from build123d import *

# Parameters (mm, degrees)
SKETCH1_R                   = 1.2
BOSS_EXTRUDE1_DEPTH         = 1.4
SKETCH2_R                   = 2.25
CUT_EXTRUDE1_DEPTH          = 1.1
CUT_EXTRUDE1_DRAFT          = -45
SKETCH3_W                   = 12
SKETCH3_H                   = 1.5
BOSS_EXTRUDE2_DEPTH         = 3.5
CIRPATTERN1_COUNT           = 2
CIRPATTERN1_ANGLE           = 90
CIRPATTERN1_COPY_1_SKETCH_R = 2.25
CIRPATTERN1_COPY_1_DEPTH    = 1.1
CIRPATTERN1_COPY_1_DRAFT    = -45
CIRPATTERN2_START           = -14
CIRPATTERN2_OUTLINE_W       = 1.5
CIRPATTERN2_OUTLINE_H       = 3.5
CIRPATTERN2_DEPTH           = 12
CIRPATTERN2_2_OUTLINE_R     = 1.2
CIRPATTERN2_2_DEPTH         = 1.4
CIRPATTERN2_START_2         = -2.1
CIRPATTERN2_3_OUTLINE_W     = 12
CIRPATTERN2_3_OUTLINE_H     = 1.5
CIRPATTERN2_3_DEPTH         = 2.1
CIRPATTERN3_COPY_1_SKETCH_R = 2.25
CIRPATTERN3_COPY_1_DEPTH    = 1.1
CIRPATTERN3_COPY_1_DRAFT    = -45
CIRPATTERN3_COPY_2_SKETCH_R = 2.25
CIRPATTERN3_COPY_2_DEPTH    = 1.1
CIRPATTERN3_COPY_2_DRAFT    = -45
CIRPATTERN3_COPY_3_SKETCH_R = 2.25
CIRPATTERN3_COPY_3_DEPTH    = 1.1
CIRPATTERN3_COPY_3_DRAFT    = -45
CUT_EXTRUDE2_DEPTH          = 3
CIRPATTERN4_COUNT           = 4
FILLET2_R                   = 0.25
CUT_EXTRUDE3_DEPTH          = 32.183489221
CUT_EXTRUDE3_DEPTH_BACK     = 32.183489221
SKETCH5_W                   = 28
SKETCH5_H                   = 28
SKETCH5_W_2                 = 27.7
SKETCH5_H_2                 = 27.7
FILLET3_R                   = 2
FILLET4_R                   = 1.1
CUT_EXTRUDE4_DEPTH          = 31.97184205
CUT_EXTRUDE4_DEPTH_BACK     = 31.97184205
SKETCH6_W                   = 0.1
SKETCH6_H                   = 2.1
CUT_EXTRUDE5_DEPTH          = 31.97184205
CUT_EXTRUDE5_DEPTH_BACK     = 31.97184205
SKETCH7_W                   = 0.1
SKETCH7_H                   = 2.1


# Read off the part's stored shape, not the designer's step: CirPattern2
with BuildPart() as part:
    # Sketch1 → Boss-Extrude1 (new body)
    with BuildSketch(Plane(origin=(0, 0, 0), x_dir=(1, 0, 0), z_dir=(0, 1, 0))):
        Polygon((0, 0), (0, 2), (-6, 2), (-6, -6), (2, -6), (2, 0), align=None)
        with Locations(Location((-2, -2, 0), (0, 0, 270))):
            Circle(SKETCH1_R, mode=Mode.SUBTRACT)
    boss_extrude1 = extrude(amount=BOSS_EXTRUDE1_DEPTH)


with BuildPart() as cut_extrude1_tool:
    # Sketch2 → Cut-Extrude1 (with draft: the straight prism first)
    with BuildSketch(Plane(origin=(0, 1.4, 0), x_dir=(1, 0, 0), z_dir=(0, 1, 0))):
        with Locations((-2, -2)):
            Circle(SKETCH2_R)
    extrude(amount=-CUT_EXTRUDE1_DEPTH)
    # Cut-Extrude1: the draft: its side faces are tilted about the plane it starts from
    cut_extrude1_sides = [cut_extrude1_tool.faces().sort_by_distance(p)[0] for p in [
        (-4.25, 0.85, 2),
    ]]
    draft(cut_extrude1_sides, Plane(origin=(0, 1.4, 0), x_dir=(1, 0, 0), z_dir=(0, 1, 0)), CUT_EXTRUDE1_DRAFT)


with BuildPart() as part_1:
    add(part.part)

    # Cut-Extrude1: cut by cut_extrude1_tool
    add(cut_extrude1_tool.part, mode=Mode.SUBTRACT)

    # Sketch3 → Boss-Extrude2 (add)
    with BuildSketch(Plane(origin=(0, 1.4, 0), x_dir=(1, 0, 0), z_dir=(0, 1, 0))):
        with Locations((8, -0.75)):
            Rectangle(SKETCH3_W, SKETCH3_H)
    boss_extrude2 = extrude(amount=-BOSS_EXTRUDE2_DEPTH)

    # CirPattern1: Boss-Extrude1, Boss-Extrude2 ×2 about axis
    cirpattern1_axis = Axis((8, 0, -8), (0, 1, 0))
    add([boss_extrude1.rotate(cirpattern1_axis, i * CIRPATTERN1_ANGLE / (CIRPATTERN1_COUNT - 1)) for i in range(1, CIRPATTERN1_COUNT)])
    add([boss_extrude2.rotate(cirpattern1_axis, i * CIRPATTERN1_ANGLE / (CIRPATTERN1_COUNT - 1)) for i in range(1, CIRPATTERN1_COUNT)])


with BuildPart() as cirpattern1_copy_1_tool:
    # CirPattern1 copy 1 sketch → CirPattern1 copy 1 (with draft: the straight prism first)
    with BuildSketch(Plane(origin=(16, 1.4, 0), x_dir=(0, 0, -1), z_dir=(0, 1, 0))):
        with Locations((-2, -2)):
            Circle(CIRPATTERN1_COPY_1_SKETCH_R)
    extrude(amount=-CIRPATTERN1_COPY_1_DEPTH)
    # CirPattern1 copy 1: the draft: its side faces are tilted about the plane it starts from
    cirpattern1_copy_1_sides = [cirpattern1_copy_1_tool.faces().sort_by_distance(p)[0] for p in [
        (18, 0.85, 4.25),
    ]]
    draft(cirpattern1_copy_1_sides, Plane(origin=(16, 1.4, 0), x_dir=(0, 0, -1), z_dir=(0, 1, 0)), CIRPATTERN1_COPY_1_DRAFT)


with BuildPart() as part_2:
    add(part_1.part)

    # CirPattern1 copy 1: cut by cirpattern1_copy_1_tool
    add(cirpattern1_copy_1_tool.part, mode=Mode.SUBTRACT)

    # CirPattern2 outline → CirPattern2 (add)
    with BuildSketch(Plane.XY.offset(CIRPATTERN2_START)):
        with Locations((-0.75, -0.35)):
            Rectangle(CIRPATTERN2_OUTLINE_W, CIRPATTERN2_OUTLINE_H)
    extrude(amount=CIRPATTERN2_DEPTH)

    # CirPattern2 2 outline → CirPattern2 2 (add)
    with BuildSketch(Plane(origin=(0, 0, 0), x_dir=(1, 0, 0), z_dir=(0, 1, 0))):
        Polygon((2, 16), (16, 16), (16, 14), (22, 14), (22, 22), (14, 22), (14, 17.5), (2, 17.5), align=None)
        with Locations((18, 18)):
            Circle(CIRPATTERN2_2_OUTLINE_R, mode=Mode.SUBTRACT)
    extrude(amount=CIRPATTERN2_2_DEPTH)

    # CirPattern2 3 outline → CirPattern2 3 (add)
    with BuildSketch(Plane(origin=(0, 0, 0), x_dir=(1, 0, 0), z_dir=(0, 1, 0)).offset(CIRPATTERN2_START_2)):
        with Locations((8, 16.75)):
            Rectangle(CIRPATTERN2_3_OUTLINE_W, CIRPATTERN2_3_OUTLINE_H)
    extrude(amount=CIRPATTERN2_3_DEPTH)

    # CirPattern2 4 outline → CirPattern2 4 (revolve)
    with BuildSketch(Plane(origin=(18, 0, 2), x_dir=(1, 0, 0), z_dir=(0, 0, 1))):
        Polygon((1.2, 1.4), (1.2, 0.35), (2.25, 1.4), align=None)
    revolve(axis=Axis((18, 0, 2), (0, 1, 0)))

    # Mirror1: Boss-Extrude1 across plane
    add(boss_extrude1.mirror(Plane(origin=(0, 0, -8), x_dir=(1, 0, 0), z_dir=(0, 0, -1))))


with BuildPart() as cirpattern3_copy_1_tool:
    # CirPattern3 copy 1 sketch → CirPattern3 copy 1 (with draft: the straight prism first)
    with BuildSketch(Plane(origin=(16, 1.4, 0), x_dir=(0, 0, -1), z_dir=(0, 1, 0))):
        with Locations((-2, -2)):
            Circle(CIRPATTERN3_COPY_1_SKETCH_R)
    extrude(amount=-CIRPATTERN3_COPY_1_DEPTH)
    # CirPattern3 copy 1: the draft: its side faces are tilted about the plane it starts from
    cirpattern3_copy_1_sides = [cirpattern3_copy_1_tool.faces().sort_by_distance(p)[0] for p in [
        (18, 0.85, 4.25),
    ]]
    draft(cirpattern3_copy_1_sides, Plane(origin=(16, 1.4, 0), x_dir=(0, 0, -1), z_dir=(0, 1, 0)), CIRPATTERN3_COPY_1_DRAFT)


with BuildPart() as part_3:
    add(part_2.part)

    # CirPattern3 copy 1: cut by cirpattern3_copy_1_tool
    add(cirpattern3_copy_1_tool.part, mode=Mode.SUBTRACT)


with BuildPart() as cirpattern3_copy_2_tool:
    # CirPattern3 copy 2 sketch → CirPattern3 copy 2 (with draft: the straight prism first)
    with BuildSketch(Plane(origin=(16, 1.4, -16), x_dir=(-1, 0, 0), z_dir=(0, 1, 0))):
        with Locations((-2, -2)):
            Circle(CIRPATTERN3_COPY_2_SKETCH_R)
    extrude(amount=-CIRPATTERN3_COPY_2_DEPTH)
    # CirPattern3 copy 2: the draft: its side faces are tilted about the plane it starts from
    cirpattern3_copy_2_sides = [cirpattern3_copy_2_tool.faces().sort_by_distance(p)[0] for p in [
        (20.25, 0.85, -18),
    ]]
    draft(cirpattern3_copy_2_sides, Plane(origin=(16, 1.4, -16), x_dir=(-1, 0, 0), z_dir=(0, 1, 0)), CIRPATTERN3_COPY_2_DRAFT)


with BuildPart() as part_4:
    add(part_3.part)

    # CirPattern3 copy 2: cut by cirpattern3_copy_2_tool
    add(cirpattern3_copy_2_tool.part, mode=Mode.SUBTRACT)


with BuildPart() as cirpattern3_copy_3_tool:
    # CirPattern3 copy 3 sketch → CirPattern3 copy 3 (with draft: the straight prism first)
    with BuildSketch(Plane(origin=(0, 1.4, -16), x_dir=(0, 0, 1), z_dir=(0, 1, 0))):
        with Locations((-2, -2)):
            Circle(CIRPATTERN3_COPY_3_SKETCH_R)
    extrude(amount=-CIRPATTERN3_COPY_3_DEPTH)
    # CirPattern3 copy 3: the draft: its side faces are tilted about the plane it starts from
    cirpattern3_copy_3_sides = [cirpattern3_copy_3_tool.faces().sort_by_distance(p)[0] for p in [
        (-2, 0.85, -20.25),
    ]]
    draft(cirpattern3_copy_3_sides, Plane(origin=(0, 1.4, -16), x_dir=(0, 0, 1), z_dir=(0, 1, 0)), CIRPATTERN3_COPY_3_DRAFT)


with BuildPart() as part_5:
    add(part_4.part)

    # CirPattern3 copy 3: cut by cirpattern3_copy_3_tool
    add(cirpattern3_copy_3_tool.part, mode=Mode.SUBTRACT)

    # Sketch4 → Cut-Extrude2 (cut)
    with BuildSketch(Plane.XY.offset(1.5)):
        with BuildLine():
            Line((6.5, 1.4), (9.5, 1.4))
            Line((9.5, 1.4), (9.5, 1.2))
            ThreePointArc((9.5, 1.2), (9.412132034, 0.987867966), (9.2, 0.9))
            Line((9.2, 0.9), (6.8, 0.9))
            ThreePointArc((6.8, 0.9), (6.587867966, 0.987867966), (6.5, 1.2))
            Line((6.5, 1.2), (6.5, 1.4))
        make_face()
    cut_extrude2 = extrude(amount=-CUT_EXTRUDE2_DEPTH, mode=Mode.SUBTRACT)

    # CirPattern4: Cut-Extrude2 ×4 about axis
    cirpattern4_axis = Axis((8, 0, -8), (0, 1, 0))
    for i in range(1, CIRPATTERN4_COUNT):
        add(cut_extrude2.rotate(cirpattern4_axis, i * 360 / CIRPATTERN4_COUNT), mode=Mode.SUBTRACT)

    # Fillet2
    fillet2_edges = [part_5.edges().sort_by_distance(p)[0] for p in [
        (6.5, 1.3, 0),
        (9.5, 1.3, 0),
        (9.412132034, 0.987867966, 0),
        (8, 0.9, 0),
        (6.587867966, 0.987867966, 0),
        (6.5, 1.3, 1.5),
        (6.587867966, 0.987867966, 1.5),
        (8, 0.9, 1.5),
        (9.412132034, 0.987867966, 1.5),
        (9.5, 1.3, 1.5),
        (16, 1.3, -6.5),
        (16, 1.3, -9.5),
        (16, 0.987867966, -9.412132034),
        (16, 0.9, -8),
        (16, 0.987867966, -6.587867966),
        (17.5, 1.3, -6.5),
        (17.5, 0.987867966, -6.587867966),
        (17.5, 0.9, -8),
        (17.5, 0.987867966, -9.412132034),
        (17.5, 1.3, -9.5),
        (9.5, 1.3, -16),
        (6.5, 1.3, -16),
        (6.587867966, 0.987867966, -16),
        (8, 0.9, -16),
        (9.412132034, 0.987867966, -16),
        (9.5, 1.3, -17.5),
        (9.412132034, 0.987867966, -17.5),
        (8, 0.9, -17.5),
        (6.587867966, 0.987867966, -17.5),
        (6.5, 1.3, -17.5),
        (0, 1.3, -9.5),
        (0, 1.3, -6.5),
        (0, 0.987867966, -6.587867966),
        (0, 0.9, -8),
        (0, 0.987867966, -9.412132034),
        (-1.5, 1.3, -9.5),
        (-1.5, 0.987867966, -9.412132034),
        (-1.5, 0.9, -8),
        (-1.5, 0.987867966, -6.587867966),
        (-1.5, 1.3, -6.5),
    ]]
    fillet(fillet2_edges, radius=FILLET2_R)

    # Sketch5 → Cut-Extrude3 (cut, two sides: drawn at the far end of the back side and taken through both)
    with BuildSketch(Plane(origin=(0, 0, 0), x_dir=(1, 0, 0), z_dir=(0, 1, 0)).offset(-CUT_EXTRUDE3_DEPTH_BACK)):
        with Locations((8, 8)):
            Rectangle(SKETCH5_W, SKETCH5_H)
        with Locations((8, 8)):
            Rectangle(SKETCH5_W_2, SKETCH5_H_2, mode=Mode.SUBTRACT)
    extrude(amount=CUT_EXTRUDE3_DEPTH + CUT_EXTRUDE3_DEPTH_BACK, mode=Mode.SUBTRACT)

    # Fillet3
    fillet3_edges = [part_5.edges().sort_by_distance(p)[0] for p in [
        (16, 0.7, -16),
        (0, 0.7, 0),
        (0, 0.7, -16),
        (16, 0.7, 0),
    ]]
    fillet(fillet3_edges, radius=FILLET3_R)

    # Fillet4
    fillet4_edges = [part_5.edges().sort_by_distance(p)[0] for p in [
        (17.5, 0.7, -14),
        (14, 0.7, -17.5),
        (-1.5, 0.7, -2),
        (-1.5, 0.7, -14),
        (2, 0.7, -17.5),
        (2, 0.7, 1.5),
        (14, 0.7, 1.5),
        (17.5, 0.7, -2),
    ]]
    fillet(fillet4_edges, radius=FILLET4_R)

    # Sketch6 → Cut-Extrude4 (cut, two sides: drawn at the far end of the back side and taken through both)
    with BuildSketch(Plane.XY.offset(-CUT_EXTRUDE4_DEPTH_BACK)):
        with Locations((13.95, -1.05)):
            Rectangle(SKETCH6_W, SKETCH6_H)
        with Locations((2.05, -1.05)):
            Rectangle(SKETCH6_W, SKETCH6_H)
    extrude(amount=CUT_EXTRUDE4_DEPTH + CUT_EXTRUDE4_DEPTH_BACK, mode=Mode.SUBTRACT)

    # Sketch7 → Cut-Extrude5 (cut, two sides: drawn at the far end of the back side and taken through both)
    with BuildSketch(Plane(origin=(0, 0, 0), x_dir=(0, 0, -1), z_dir=(1, 0, 0)).offset(-CUT_EXTRUDE5_DEPTH_BACK)):
        with Locations((2.05, -1.05)):
            Rectangle(SKETCH7_W, SKETCH7_H)
        with Locations((13.95, -1.05)):
            Rectangle(SKETCH7_W, SKETCH7_H)
    extrude(amount=CUT_EXTRUDE5_DEPTH + CUT_EXTRUDE5_DEPTH_BACK, mode=Mode.SUBTRACT)


solid = part_5.part
Verification items for the finished model (mm, model axes). A direction names the side the tool comes from. Coordinates: 2 decimals unless noted, no trailing zeros. Order: outer loops, then holes, each group sorted by start corner. A loop starts at its lowest first (then second) coordinate and runs counter-clockwise, first axis right, second up. Notation, with made-up numbers: M -35.5,-36.5 L 23.5,-36.5 A6 ccw 23.5,-25.5 Z; hole C -15.5,60 d3. An arc over 180 degrees is marked long. One line per item, written item: value. Start each with the question number.
Item 1: Scan lines: probe 1 along X at (y, z) = (0.4, -10.25); probe 2 along Z at (x, y) = (-2, 0.3); probe 3 along Z at (x, y) = (10.75, -0.65). Record each from-to range of solid material in increasing order.
Item 2: Mould release check, pull along Z, two halves, no side actions. Record for faces 3 (the flat face through (17, -2.1, -8)), 4 (the flat face through (-2, 1, 5.85)), 5 (the flat face through (-1, 0.9, -8)): released by +Z, released by -Z, zero draft, split by the parting line, or undercut.
Item 3: Sectioned sample at C-C (x = 0.75). Enter the section's corners in (y, z), then the cut area to 3 significant figures.
Item 4: Gauge pin test, flat ends, axial feed: pin 1 (4 mm diameter, centred on x = 18, z = -18, fed in from -Y); pin 2 (2 mm diameter, centred on y = -1.5, z = -14, fed in from -X); pin 3 (1 mm diameter, centred on x = 12, y = -1, fed in from +Z); pin 4 (1.7 mm diameter, centred on y = -0.5, z = 1, fed in from -X). Record the tip position at first contact, or that the pin passes through.
Item 5: Sectioned sample at B-B (y = -0.8). Enter the section's corners in (x, z).
Item 6: Sectioned sample at A-A (z = -5.75). Enter the section's corners in (x, y).
Item 7: Sectioned sample at D-D (z = -18). Enter the section's corners in (x, y).
Item 8: Access from +Z, -Z, +X, -X, +Y, -Y to the whole of each face (thin tool, end or side, straight path). Record for faces 1 (the flat face through (13.9, -1, -17)), 2 (the flat face through (20, 1, -14)).
Conclusion:
1. probe 1: x = -1.5 to 0, 16 to 17.5
1. probe 2: z = -21.85 to -19.2, -16.8 to -13.82, -2.18 to 0.8, 3.2 to 5.85
1. probe 3: z = -17.5 to -16, 0 to 1.5
2. face 3: zero draft
2. face 4: released by +Z
2. face 5: undercut
3. outline: M 0,-21.85 L 1.4,-21.85 L 1.4,-15.56 L 0,-15.56 Z; M 0,-0.44 L 1.4,-0.44 L 1.4,5.85 L 0,5.85 Z
3. area: 17.6 mm^2
4. pin 1: stops at y = 0
4. pin 2: stops at x = -1.5
4. pin 3: stops at z = 1.5
4. pin 4: stops at x = -5.85
5. outline: M -1.5,-13.9 L 0,-13.9 L 0,-2.1 L -1.5,-2.1 Z; M 2.1,-17.5 L 13.9,-17.5 L 13.9,-16 L 2.1,-16 Z; M 2.1,0 L 13.9,0 L 13.9,1.5 L 2.1,1.5 Z; M 16,-13.9 L 17.5,-13.9 L 17.5,-2.1 L 16,-2.1 Z
6. outline: M -1.5,-2.1 L 0,-2.1 L 0,1.4 L -1.5,1.4 Z; M 16,-2.1 L 17.5,-2.1 L 17.5,1.4 L 16,1.4 Z
7. outline: M -5.85,0 L -3.2,0 L -3.2,0.35 L -4.25,1.4 L -5.85,1.4 Z; M -0.8,0 L 2.18,0 L 2.18,1.4 L 0.25,1.4 L -0.8,0.35 Z; M 13.82,0 L 16.8,0 L 16.8,0.35 L 15.75,1.4 L 13.82,1.4 Z; M 19.2,0 L 21.85,0 L 21.85,1.4 L 20.25,1.4 L 19.2,0.35 Z
8. face 1: +Z, -Z, +X, -Y
8. face 2: +X, +Y, -Y
